The listing builds one solid part. Answer for the finished solid, in the listing's coordinates (mm). Face numbers are marked on the shaded views. Coordinates: 2 decimals unless noted, no trailing zeros. Write each loop counter-clockwise with the first axis right and the second up, starting at its lowest first coordinate (ties: lowest second). Pieces come first, ordered by that corner, then holes.
(1) The part is cut by section B-B on z = 3. Determine the outline of the cut face in (x, y), plus the area to 3 significant figures.
(2) Straight lines are drawn through the part: line 1 (X direction, y = -12, z = 2); line 2 (X direction, y = -20.75, z = 13.5); line 3 (Z direction, x = -1.5, y = -1.25). For each, find the intervals that lie inside material, in ascending order.
(3) Given P1, Ø1.5, axis at x = 25.5, y = -23, coming from the +Z side; P2, Ø1, axis at y = -21, z = 10, coming from the -X side; P3, Ø4, axis at y = -21, z = 0.5, coming from the +X side, each flat-ended and moving along its own axis, determine where each tip first touches the part or whether it passes through.
(4) The part is cut by section A-A on x = -2. Determine the outline of the cut face in (y, z), plus the area to 3 significant figures.
(5) The part is cut by section D-D on y = -3. Determine the outline of the cut face in (x, z), plus the area to 3 significant figures.
(6) For a pull along Z with two mould halves and no side action, classify the marked faces 1, 2, 3 and 4 as +Z half, -Z half, draft (parallel to the pull), parting line (faces both ways), or undercut.
(7) The part is cut by section C-C on x = 33. Determine the outline of the cut face in (y, z).
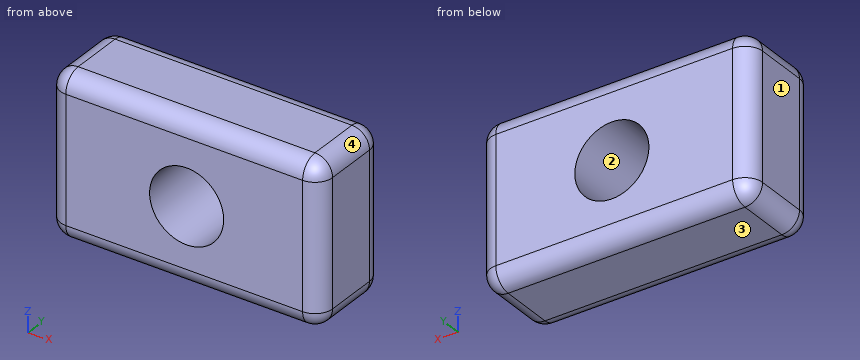
from build123d import *

# Parameters (mm, degrees)
F0_W         = 78.3818922937
F0_H         = 46.5174447745
F1_DEPTH     = 25.4
F2_R         = 5.08
F3_T1_DEPTH  = 15.24
F3_S5_W      = 5.08
F3_S5_H      = 5.08
F3_T6_DEPTH  = 5.08
F3_S11_W     = 5.08
F3_S11_H     = 5.08
F3_T12_DEPTH = 5.08
F4_R         = 10.6653295048
F5_DEPTH     = 25.4


# Not quite as in the source:
# - a fillet or chamfer that OpenCascade refuses, or shapes differently, is made with other operations: its cross-section is extruded or revolved along the edge and cut away or added


with BuildPart() as f1:
    # F0 (on Front) → F1 (new body)
    with BuildSketch(Plane.XZ):
        with Locations((1.8606986851, 2.9073404148)):
            Rectangle(F0_W, F0_H)
    extrude(amount=F1_DEPTH)

    # F2
    f2_edges = [f1.edges().sort_by_distance(p)[0] for p in [
        (41.051645, -12.7, 26.166063),
        (1.860699, -25.4, 26.166063),
        (1.860699, 0, 26.166063),
        (41.051645, -25.4, 2.90734),
        (41.051645, 0, 2.90734),
        (-37.330247, 0, 2.90734),
        (1.860699, 0, -20.351382),
        (41.051645, -12.7, -20.351382),
        (-37.330247, -12.7, -20.351382),
        (-37.330247, -25.4, 2.90734),
        (1.860699, -25.4, -20.351382),
    ]]
    fillet(f2_edges, radius=F2_R)

    # F3: fillet of radius 5.08 on 1 edges, made by hand

    # F3_s2 → F3_t1 (cut)
    with BuildSketch(Plane.XZ.offset(5.08)):
        with BuildLine():
            ThreePointArc((-32.2502474618, 26.1660628021), (-35.8423499102, 24.6781652505), (-37.3302474618, 21.0860628021))
            Line((-37.3302474618, 21.0860628021), (-37.3302474618, 26.1660628021))
            Line((-37.3302474618, 26.1660628021), (-32.2502474618, 26.1660628021))
        make_face()
    extrude(amount=F3_T1_DEPTH, mode=Mode.SUBTRACT)


with BuildPart() as f3_tool4:
    # F3_s5 → F3_t6 (new body)
    with BuildSketch(Plane.XY.offset(21.0860628021)):
        with Locations((-34.7902474618, -2.54)):
            Rectangle(F3_S5_W, F3_S5_H)
    extrude(amount=F3_T6_DEPTH)

    # F3_s7 → F3_t8 (revolve, cut)
    with BuildSketch(Plane(origin=(-32.2502474618, -5.08, 21.0860628021), x_dir=(0.7071067812, -0.7071067812, 0), z_dir=(-0.7071067812, -0.7071067812, 0))):
        with BuildLine():
            ThreePointArc((0, -5.08), (5.08, 0), (0, 5.08))
            Line((0, 5.08), (0, -5.08))
        make_face()
    revolve(axis=Axis((-32.2502474618, -5.08, 21.0860628021), (0, 0, 1)), mode=Mode.SUBTRACT)


with BuildPart() as f1_1:
    add(f1.part)

    # F3_t3: cut F3_tool4
    add(f3_tool4.part, mode=Mode.SUBTRACT)


with BuildPart() as f3_tool10:
    # F3_s11 → F3_t12 (new body)
    with BuildSketch(Plane.XY.offset(21.0860628021)):
        with Locations((-34.7902474618, -22.86)):
            Rectangle(F3_S11_W, F3_S11_H)
    extrude(amount=F3_T12_DEPTH)

    # F3_s13 → F3_t14 (revolve, cut)
    with BuildSketch(Plane(origin=(-32.2502474618, -20.32, 21.0860628021), x_dir=(0.7071067812, 0.7071067812, 0), z_dir=(0.7071067812, -0.7071067812, 0))):
        with BuildLine():
            ThreePointArc((0, -5.08), (5.08, 0), (0, 5.08))
            Line((0, 5.08), (0, -5.08))
        make_face()
    revolve(axis=Axis((-32.2502474618, -20.32, 21.0860628021), (0, 0, 1)), mode=Mode.SUBTRACT)


with BuildPart() as f1_2:
    add(f1_1.part)

    # F3_t9: cut F3_tool10
    add(f3_tool10.part, mode=Mode.SUBTRACT)

    # F4 (on face) → F5 (cut, through all)
    with BuildSketch(Plane.XZ.offset(25.4)):
        with Locations((2.5458505843, 2.2031988483)):
            Circle(F4_R)
    extrude(amount=-F5_DEPTH, mode=Mode.SUBTRACT)


solid = f1_2.part
Model answer:
1. outline: (-37.33, -20.32) arc R5.08 ccw to (-32.25, -25.4) - (-8.09, -25.4) - (-8.09, 0) - (-32.25, 0) arc R5.08 ccw to (-37.33, -5.08) - close; (13.18, -25.4) - (35.97, -25.4) arc R5.08 ccw to (41.05, -20.32) - (41.05, -5.08) arc R5.08 ccw to (35.97, 0) - (13.18, 0) - close
1. area: 1,430 mm2
2. line 1: x = -37.33 to -8.12, 13.21 to 41.05
2. line 2: x = -37.31 to 41.03
2. line 3: z = -18.61 to -7.66, 12.07 to 24.42
3. P1: stops at z = 25.79
3. P2: stops at x = -37.33
3. P3: stops at x = 41.05
4. outline: (-25.4, -15.27) arc R5.08 ccw to (-20.32, -20.35) - (-5.08, -20.35) arc R5.08 ccw to (0, -15.27) - (0, -7.44) - (-25.4, -7.44) - close; (-25.4, 11.85) - (0, 11.85) - (0, 21.09) arc R5.08 ccw to (-5.08, 26.17) - (-20.32, 26.17) arc R5.08 ccw to (-25.4, 21.09) - close
4. area: 669 mm2
5. outline: (-36.88, -15.27) arc R4.63 ccw to (-32.25, -19.91) - (35.97, -19.91) arc R4.63 ccw to (40.61, -15.27) - (40.61, 21.09) arc R4.63 ccw to (35.97, 25.72) - (-32.25, 25.72) arc R4.63 ccw to (-36.88, 21.09) - close; hole circle Ø21.33 at (2.55, 2.2)
5. area: 3,160 mm2
6. face 1: draft
6. face 2: undercut
6. face 3: -Z half
6. face 4: +Z half
7. outline: (-25.4, -15.27) arc R5.08 ccw to (-20.32, -20.35) - (-5.08, -20.35) arc R5.08 ccw to (0, -15.27) - (0, 21.09) arc R5.08 ccw to (-5.08, 26.17) - (-20.32, 26.17) arc R5.08 ccw to (-25.4, 21.09) - close
